The model under review builds one solid part; all positions refer to its coordinate system, in mm. Face numbers are marked on the shaded views. A direction names the side the tool comes from. Coordinates: 2 decimals unless noted, no trailing zeros. Loops run counter-clockwise (first coordinate to the right, second up) from the corner with the lowest first, then second, coordinate; pieces in that order, holes last. Notation, with made-up numbers: M -23,-1.5 L -12,-1.5 A22 ccw -12,25.5 Z; hole C -24,77 d2. An arc over 180 degrees is marked long. Return JSON: item names as keys, results as strings.
```python
from build123d import *

# Parameters (mm, degrees)
SKETCH2_R           = 2.5
BOSS_EXTRUDE2_DEPTH = 30


with BuildPart() as part:
    # Sketch2 → Boss-Extrude2 (new body)
    with BuildSketch(Plane(origin=(0, 0, 0), x_dir=(0, 0, -1), z_dir=(1, 0, 0))):
        with BuildLine():
            Line((30.085747665, -11.186099671), (21.541651222, -15.763294195))
            ThreePointArc((21.541651222, -15.763294195), (19.517636628, -17.343724655), (18.545040528, -19.720371945))
            Line((18.545040528, -19.720371945), (18.545040528, -25.085535704))
            ThreePointArc((18.545040528, -25.085535704), (19.410646287, -26.94173637), (20.947854528, -28.295156137))
            Line((20.947854528, -28.295156137), (29.255531223, -32.745697224))
            ThreePointArc((29.255531223, -32.745697224), (30.70940007, -33.921076219), (31.629897073, -35.548324102))
            ThreePointArc((31.629897073, -35.548324102), (32.071931866, -36.783630966), (32.555458455, -38.00329479))
            ThreePointArc((32.555458455, -38.00329479), (32.932855534, -39.672508554), (32.725254973, -41.37121546))
            Line((32.725254973, -41.37121546), (30.127327196, -49.964361184))
            ThreePointArc((30.127327196, -49.964361184), (29.813665847, -52.513088724), (30.806479965, -54.881361437))
            Line((30.806479965, -54.881361437), (34.600223641, -58.675105113))
            ThreePointArc((34.600223641, -58.675105113), (36.524831421, -59.37556149), (38.568814087, -59.245603413))
            Line((38.568814087, -59.245603413), (46.247135524, -56.924250421))
            ThreePointArc((46.247135524, -56.924250421), (48.189416877, -56.734903616), (50.056242855, -57.303471848))
            ThreePointArc((50.056242855, -57.303471848), (52.14714523, -58.344514128), (54.296872356, -59.257922611))
            ThreePointArc((54.296872356, -59.257922611), (55.797855342, -60.175122269), (56.888305405, -61.555384489))
            Line((56.888305405, -61.555384489), (60.38212329, -68.077177874))
            ThreePointArc((60.38212329, -68.077177874), (61.96255375, -70.101192468), (64.339201041, -71.073788567))
            Line((64.339201041, -71.073788567), (69.7043648, -71.073788567))
            ThreePointArc((69.7043648, -71.073788567), (71.560565466, -70.208182809), (72.913985233, -68.670974568))
            Line((72.913985233, -68.670974568), (76.025985896, -62.861906663))
            ThreePointArc((76.025985896, -62.861906663), (77.294737312, -61.33085674), (79.059877782, -60.415366082))
            ThreePointArc((79.059877782, -60.415366082), (82.213367183, -59.366491991), (85.265589491, -58.05174059))
            ThreePointArc((85.265589491, -58.05174059), (87.048884387, -57.57014809), (88.885340547, -57.768896167))
            Line((88.885340547, -57.768896167), (94.58319028, -59.4915019))
            ThreePointArc((94.58319028, -59.4915019), (97.13191782, -59.805163248), (99.500190533, -58.812349131))
            Line((99.500190533, -58.812349131), (103.293934209, -55.018605455))
            ThreePointArc((103.293934209, -55.018605455), (103.994390585, -53.093997675), (103.864432509, -51.050015008))
            Line((103.864432509, -51.050015008), (102.151862248, -45.385359528))
            ThreePointArc((102.151862248, -45.385359528), (101.963471996, -43.433562355), (102.540152369, -41.559411123))
            ThreePointArc((102.540152369, -41.559411123), (104.144447245, -38.22268307), (105.423574244, -34.748298193))
            ThreePointArc((105.423574244, -34.748298193), (106.342936692, -33.05955411), (107.831618895, -31.842627988))
            Line((107.831618895, -31.842627988), (112.696006969, -29.236705805))
            ThreePointArc((112.696006969, -29.236705805), (114.720021563, -27.656275345), (115.692617663, -25.279628055))
            Line((115.692617663, -25.279628055), (115.692617663, -19.914464296))
            ThreePointArc((115.692617663, -19.914464296), (114.827011904, -18.05826363), (113.289803663, -16.704843863))
            Line((113.289803663, -16.704843863), (107.614484835, -13.664494491))
            ThreePointArc((107.614484835, -13.664494491), (106.151590865, -12.478432267), (105.231215931, -10.835352127))
            ThreePointArc((105.231215931, -10.835352127), (104.073253902, -7.788047033), (102.663702949, -4.848640544))
            ThreePointArc((102.663702949, -4.848640544), (102.101264993, -2.987400021), (102.291326141, -1.05234718))
            Line((102.291326141, -1.05234718), (104.110330995, 4.964361184))
            ThreePointArc((104.110330995, 4.964361184), (104.423992344, 7.513088724), (103.431178226, 9.881361437))
            Line((103.431178226, 9.881361437), (99.63743455, 13.675105113))
            ThreePointArc((99.63743455, 13.675105113), (97.71282677, 14.375561489), (95.668844104, 14.245603413))
            Line((95.668844104, 14.245603413), (88.104104481, 11.958589109))
            ThreePointArc((88.104104481, 11.958589109), (86.316773657, 11.75624578), (84.573495165, 12.199500102))
            ThreePointArc((84.573495165, 12.199500102), (82.504544688, 13.07643575), (80.388319531, 13.832189213))
            ThreePointArc((80.388319531, 13.832189213), (78.725157037, 14.752239447), (77.525530925, 16.22651863))
            Line((77.525530925, 16.22651863), (73.855534901, 23.077177874))
            ThreePointArc((73.855534901, 23.077177874), (72.275104441, 25.101192468), (69.89845715, 26.073788567))
            Line((69.89845715, 26.073788567), (64.533293391, 26.073788567))
            ThreePointArc((64.533293391, 26.073788567), (62.677092726, 25.208182809), (61.323672958, 23.670974568))
            Line((61.323672958, 23.670974568), (56.878792468, 15.373864318))
            ThreePointArc((56.878792468, 15.373864318), (55.788778276, 13.99398857), (54.288444878, 13.076825711))
            ThreePointArc((54.288444878, 13.076825711), (53.130789266, 12.603622826), (51.988977307, 12.093374908))
            ThreePointArc((51.988977307, 12.093374908), (50.232381905, 11.637586716), (48.428806148, 11.838794991))
            Line((48.428806148, 11.838794991), (39.654467911, 14.4915019))
            ThreePointArc((39.654467911, 14.4915019), (37.105740371, 14.805163248), (34.737467658, 13.812349131))
            Line((34.737467658, 13.812349131), (30.943723982, 10.018605455))
            ThreePointArc((30.943723982, 10.018605455), (30.243267606, 8.093997675), (30.373225682, 6.050015008))
            Line((30.373225682, 6.050015008), (33.27387934, -3.544454783))
            ThreePointArc((33.27387934, -3.544454783), (33.476910751, -5.321546901), (33.041482883, -7.056390042))
            ThreePointArc((33.041482883, -7.056390042), (32.694654044, -7.844321785), (32.365382945, -8.639750737))
            ThreePointArc((32.365382945, -8.639750737), (31.449885158, -10.113748997), (30.085747665, -11.186099671))
        make_face()
        with Locations((67.118829096, -22.5)):
            Circle(SKETCH2_R, mode=Mode.SUBTRACT)
    extrude(amount=BOSS_EXTRUDE2_DEPTH)


solid = part.part
```
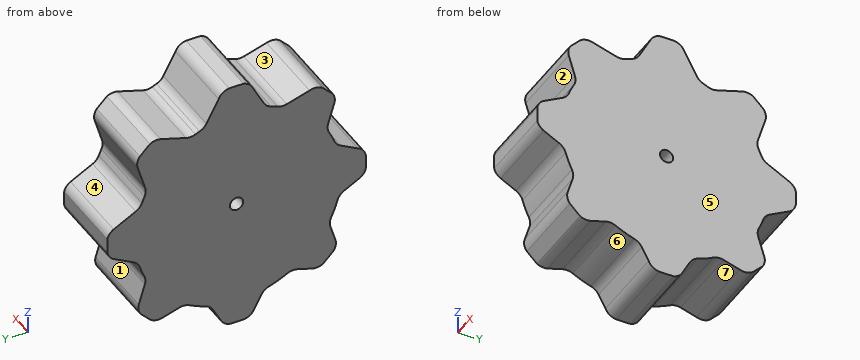
1. Add section B-B on z = -45. Give the boundary of the cut face in (x, y), plus the area to 3 significant figures.
Check values:
{"outline": "M 0,-57.3 L 30,-57.3 L 30,12.88 L 0,12.88 Z", "area": "2,110 mm²"}
2. To check wall thickness, follow line 1 (Y direction, x = 13.75, z = -96.5); line 2 (Y direction, x = 2.5, z = -61); line 3 (Z direction, x = 9.5, y = -28). State the ranges of each line that lie inside material, in increasing order.
Check values:
{"line 1": "-59.85 to 14.4", "line 2": "-69.14 to 23.07", "line 3": "-114.43 to -20.49"}
3. Add section A-A on y = -22.5. Give the boundary of the cut face in (x, z).
Check values:
{"outline": "M 0,-115.69 L 30,-115.69 L 30,-69.62 L 0,-69.62 Z; M 0,-64.62 L 30,-64.62 L 30,-18.55 L 0,-18.55 Z"}
4. Machinability: for the marked faces 1, 2 and 3, which of the approach directions +Z, -Z, +X, -X, +Y, -Y give a long, thin tool a straight path to every point of the face, cutting with its end or side? Answer none if there is none.
Check values:
{"face 1": "+X, -X, +Y", "face 2": "+X, -X, -Y", "face 3": "+Z, +X, -X"}
5. Insertion check: pin 1 Ø1 at (x, z) = (25, -87.5) entering from +Y; pin 2 Ø6 at (x, y) = (9, -53) entering from +Z; pin 3 Ø1.5 at (x, y) = (22, -12.5) entering from -Z; pin 4 Ø3 at (y, z) = (-22.5, -67.12) entering from +X. Each pin has a flat end and moves straight along its axis. Give the tip position at first contact, or say it passes through.
Check values:
{"pin 1": "y = 11.93", "pin 2": "z = -29.77", "pin 3": "z = -106.97", "pin 4": "through"}
6. The part is to be moulded in two halves that separate along Y. For the marked faces 4, 5, 6 and 7, say which applies: released by +Y, released by -Y, zero draft, split by the parting line, or undercut.
Check values:
{"face 4": "released by +Y", "face 5": "zero draft", "face 6": "undercut", "face 7": "undercut"}
